from build123d import *

# Parameters (mm, degrees)
CUT_EXTRUDE1_DEPTH                   = 159.216212497
CUT_EXTRUDE1_DEPTH_BACK              = 159.216212497
CUT_REVOLVE1_ANGLE                   = 45
CUT_EXTRUDE2_DEPTH                   = 138.24977239
CUT_EXTRUDE2_DEPTH_BACK              = 138.24977239
CUT_EXTRUDE3_DEPTH                   = 138.24977239
CUT_EXTRUDE3_DEPTH_BACK              = 138.24977239
CUT_EXTRUDE4_DEPTH                   = 138.24977239
CUT_EXTRUDE4_DEPTH_BACK              = 138.24977239
SKETCH6_R                            = 13.75
F_10_0_10_DIAMETER_HOLE1_D           = 10
F_10_0_10_DIAMETER_HOLE1_DEPTH       = 10
F_10_0_10_DIAMETER_HOLE1_CSINK_D     = 10.05
F_10_0_10_DIAMETER_HOLE1_CSINK_ANGLE = 90
CIRPATTERN1_COUNT                    = 6
FILLET3_R                            = 10
FILLET4_R                            = 5


with BuildPart() as part:
    # Sketch1 → Revolve1 (revolve)
    with BuildSketch(Plane.XY, mode=Mode.PRIVATE) as revolve1_sk:
        Polygon((0, 0), (-62.5, 0), (-62.5, 10), (-37.5, 10), (-37.5, 25), (-83.688021535, 105), (0, 105), align=None)
    revolve(revolve1_sk.sketch.rotate(Axis((0, 0, 0), (0, 1, 0)), 270), axis=Axis((0, 0, 0), (0, 1, 0)))

    # Sketch2 → Cut-Extrude1 (cut, two sides: drawn at the far end of the back side and taken through both)
    with BuildSketch(Plane(origin=(0, 0, 0), x_dir=(0, 0, -1), z_dir=(1, 0, 0)).offset(-CUT_EXTRUDE1_DEPTH_BACK)):
        with BuildLine():
            Line((-24.573687175, 84.59716202), (-31.233944355, 23.782787827))
            ThreePointArc((-31.233944355, 23.782787827), (-33.891761116, 20.167448423), (-37.5, 17.5))
            Line((-37.5, 17.5), (-101.023811283, 17.5))
            Line((-101.023811283, 17.5), (-101.023811283, 124.521875929))
            Line((-101.023811283, 124.521875929), (93.829847102, 124.521875929))
            Line((93.829847102, 124.521875929), (93.829847102, 17.5))
            Line((93.829847102, 17.5), (37.5, 17.5))
            ThreePointArc((37.5, 17.5), (33.891761116, 20.167448423), (31.233944355, 23.782787827))
            Line((31.233944355, 23.782787827), (24.573687175, 84.59716202))
            ThreePointArc((24.573687175, 84.59716202), (0, 105), (-24.573687175, 84.59716202))
        make_face()
    extrude(amount=CUT_EXTRUDE1_DEPTH + CUT_EXTRUDE1_DEPTH_BACK, mode=Mode.SUBTRACT)

    # Sketch3 → Cut-Revolve1 (revolve, symmetric, cut)
    with BuildSketch(Plane.XY) as cut_revolve1_sk:
        Polygon((47.5, 105), (43.500508947, 28.685164541), (102.973812388, 28.685164541), (102.973812388, 105), align=None)
    cut_revolve1 = revolve(axis=Axis((-52.5, 30.66973461, 0), (0, 1, 0)), revolution_arc=CUT_REVOLVE1_ANGLE / 2, mode=Mode.SUBTRACT)
    cut_revolve1 = cut_revolve1 + revolve(cut_revolve1_sk.sketch, axis=Axis((-52.5, 30.66973461, 0), (0, -1, 0)), revolution_arc=CUT_REVOLVE1_ANGLE / 2, mode=Mode.SUBTRACT)

    # Mirror1: Cut-Revolve1 across plane
    add(cut_revolve1.mirror(Plane(origin=(0, 0, 0), x_dir=(0, 0, 1), z_dir=(1, 0, 0))), mode=Mode.SUBTRACT)

    # Sketch4 → Cut-Extrude2 (cut, two sides: drawn at the far end of the back side and taken through both)
    with BuildSketch(Plane.XY.offset(-CUT_EXTRUDE2_DEPTH_BACK)):
        Polygon((-32.197983939, 105), (-22.5, 50), (22.5, 50), (32.197983939, 105), align=None)
    extrude(amount=CUT_EXTRUDE2_DEPTH + CUT_EXTRUDE2_DEPTH_BACK, mode=Mode.SUBTRACT)

    # Sketch5 → Cut-Extrude3 (cut, two sides: drawn at the far end of the back side and taken through both)
    with BuildSketch(Plane.XY.offset(-CUT_EXTRUDE3_DEPTH_BACK)):
        Polygon((37.697983939, 105), (32.197983939, 105), (29.553079228, 90), align=None)
        Polygon((-29.553079228, 90), (-37.697983939, 105), (-32.197983939, 105), align=None)
    extrude(amount=CUT_EXTRUDE3_DEPTH + CUT_EXTRUDE3_DEPTH_BACK, mode=Mode.SUBTRACT)

    # Sketch6 → Cut-Extrude4 (cut, two sides: drawn at the far end of the back side and taken through both)
    with BuildSketch(Plane(origin=(0, 0, 0), x_dir=(0, 0, -1), z_dir=(1, 0, 0)).offset(-CUT_EXTRUDE4_DEPTH_BACK)):
        with Locations(Location((0, 80, 0), (0, 0, 315.504858884))):
            Circle(SKETCH6_R)
    extrude(amount=CUT_EXTRUDE4_DEPTH + CUT_EXTRUDE4_DEPTH_BACK, mode=Mode.SUBTRACT)

    # Ø10.0 (10) Diameter Hole1
    with Locations(Plane(origin=(0, 10, 0), x_dir=(1, 0, 0), z_dir=(0, 1, 0))):
        with Locations((0, 52.5)):
            f_10_0_10_diameter_hole1 = CounterSinkHole(F_10_0_10_DIAMETER_HOLE1_D / 2, F_10_0_10_DIAMETER_HOLE1_CSINK_D / 2, depth=F_10_0_10_DIAMETER_HOLE1_DEPTH, counter_sink_angle=F_10_0_10_DIAMETER_HOLE1_CSINK_ANGLE)

    # CirPattern1: Ø10.0 (10) Diameter Hole1 ×6 about axis
    cirpattern1_axis = Axis((0, 0, 0), (0, 1, 0))
    for i in range(1, CIRPATTERN1_COUNT):
        add(f_10_0_10_diameter_hole1.rotate(cirpattern1_axis, i * 360 / CIRPATTERN1_COUNT), mode=Mode.SUBTRACT)

    # Fillet3
    fillet3_edges = [part.edges().sort_by_distance(p)[0] for p in [
        (22.5, 50, 0),
        (-22.5, 50, 0),
    ]]
    fillet(fillet3_edges, radius=FILLET3_R)

    # Fillet4
    fillet4_edges = [part.edges().sort_by_distance(p)[0] for p in [
        (0, 10, 37.5),
    ]]
    fillet(fillet4_edges, radius=FILLET4_R)


solid = part.part
Verification items for the finished model (mm, model axes). A direction names the side the tool comes from. Give positions to 0.01 mm unless a question says otherwise; leave off trailing zeros. Write each loop counter-clockwise with the first axis right and the second up, starting at its lowest first coordinate (ties: lowest second). Pieces come first, ordered by that corner, then holes.
(1) Material ranges on line 1 (Z direction, x = -0.5, y = 4); line 2 (X direction, y = 7.25, z = -26.25); line 3 (Y direction, x = -35.5, z = 34), recorded low to high.
(2) Cross-section at C-C (y = 28). Enter the section's corners in (x, z).
(3) Access from +Z, -Z, +X, -X, +Y, -Y to the whole of each face (thin tool, end or side, straight path). Record for faces 5 (the face through (40.859, 30.825, 0.559)), 6 (the face through (25.472, 66.857, 5.717)), 7 (the face through (41, 10, -13)).
(4) Mould release check, pull along Y, two halves, no side actions. Record for faces 1 (the face through (-0.651, 4.918, 57.457)), 2 (the face through (45.266, 62.389, 0.414)), 3 (the face through (33.57, 97.4, -0.32)), 4 (the face through (-1.649, 16.737, 37.464)): +Y half, -Y half, draft (parallel to the pull), parting line (faces both ways), or undercut.
(5) Cross-section at B-B (z = -52.5). Enter the section's corners in (x, y) (3 decimals), plus the area to 3 significant figures.
(6) Gauge pin test, flat ends, axial feed: pin 1 (9 mm diameter, centred on x = -45.47, z = 26.25, fed in from +Y); pin 2 (11.5 mm diameter, centred on x = 0, z = 52.5, fed in from +Y); pin 3 (4 mm diameter, centred on y = 77.5, z = 13.5, fed in from -X). Record the tip position at first contact, or that the pin passes through.
(7) Cross-section at A-A (x = 0). State how many separate pieces and enclosed holes the cut face has, plus the area to 3 significant figures.
Worked out:
1. line 1: z = -62.5 to -57.47, -47.53 to 47.53, 57.47 to 62.5
1. line 2: x = -56.72 to -50.47, -40.47 to 40.47, 50.47 to 56.72
1. line 3: y = 0 to 10
2. outline: (-24.34, -30.77) - (24.34, -30.77) arc R39.23 ccw to (24.34, 30.77) - (-24.34, 30.77) arc R39.23 ccw to start
3. face 5: +X
3. face 6: +Z, -Z, +Y
3. face 7: none
4. face 1: draft
4. face 2: undercut
4. face 3: +Y half
4. face 4: undercut
5. outline: (-33.912, 0) - (-5, 0) - (-5, 9.975) - (-5.025, 10) - (-33.912, 10) - close; (5, 0) - (33.912, 0) - (33.912, 10) - (5.025, 10) - (5, 9.975) - close
5. area: 578 mm2
6. pin 1: stops at y = 92.09
6. pin 2: stops at y = 10
6. pin 3: stops at x = -45.2
7. separate pieces: 3
7. enclosed holes: 0
7. area: 3,610 mm2
